```python
from build123d import *

# Parameters (mm, degrees)
BOSS_EXTRUDE1_DEPTH = 8.89
SKETCH3_R           = 3.556
BOSS_EXTRUDE2_DEPTH = 3.556


with BuildPart() as part:
    # Sketch2 → Boss-Extrude1 (new body)
    with BuildSketch(Plane.XY):
        with BuildLine():
            Line((-22.184810127, 0), (-33.106810127, 0))
            Line((-33.106810127, 0), (-33.106810127, 7.62))
            Line((-33.106810127, 7.62), (-25.486810127, 7.62))
            ThreePointArc((-25.486810127, 7.62), (-6.944810127, 22.300018764), (11.597189873, 7.62))
            Line((11.597189873, 7.62), (19.217189873, 7.62))
            Line((19.217189873, 7.62), (19.217189873, 0))
            Line((19.217189873, 0), (8.295189873, 0))
            ThreePointArc((8.295189873, 0), (-6.944810127, 15.24), (-22.184810127, 0))
        make_face()
    extrude(amount=BOSS_EXTRUDE1_DEPTH)

    # Sketch3 → Boss-Extrude2 (add)
    with BuildSketch(Plane.XZ):
        with Locations(Location((-27.645810127, 4.445, 0), (0, 0, 90))):
            Circle(SKETCH3_R)
        with Locations(Location((13.756189873, 4.445, 0), (0, 0, 90))):
            Circle(SKETCH3_R)
    extrude(amount=BOSS_EXTRUDE2_DEPTH)


solid = part.part
```
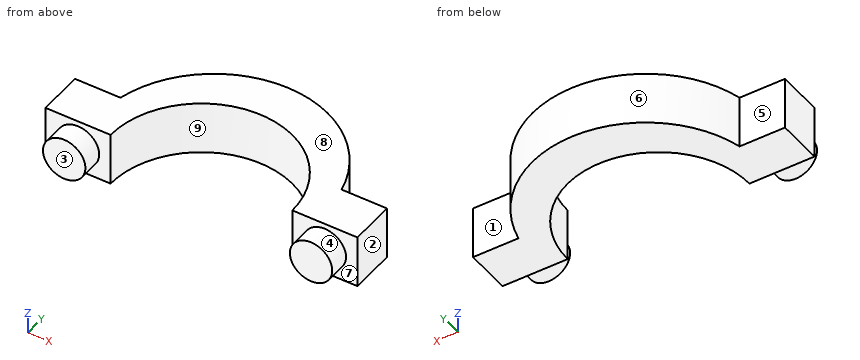
Geometry: final body of the model. Coordinates: model frame, mm. Face numbers are marked on the shaded views. A direction names the side the tool comes from. Round coordinates to 2 decimals unless told otherwise and drop trailing zeros. Write each loop counter-clockwise with the first axis right and the second up, starting at its lowest first coordinate (ties: lowest second). Pieces come first, ordered by that corner, then holes.
Item 1: Mould query, pull axis X, two halves, no side actions, for the marked faces 6, 7, 8 and 9. Classes: +X half, -X half, draft (parallel to the pull), parting line (faces both ways), or undercut.
Item 2: Section query C-C (y = 10). Return loops of the section in (x, z).
Item 3: Set-up query: the marked faces 1, 2, 3, 4 and 5. Return all of +Z, -Z, +X, -X, +Y, -Y with unobstructed straight access to the full face (end or side cutting, diameter ignored); none if empty.
Item 4: Material intervals for L1, parallel to X at y = -2, z = 6.5; L2, parallel to X at y = -2.5, z = 2.75; L3, parallel to Y at x = -28, z = 4.75, sorted ascending.
Item 5: Pin query (flat end, axial travel): P1, Ø4, axis at x = -28, z = 4, coming from the +Y side; P2, Ø8, axis at x = -3.5, y = 17, coming from the -Z side; P3, Ø3, axis at x = -8, y = 12, coming from the -Z side; P4, Ø4, axis at x = 10.5, z = 3, coming from the +Y side. Return the tip coordinate at first contact, or that it passes through.
Item 6: Section query A-A (y = 14). Return loops of the section in (x, z), plus the area to 3 significant figures.
Item 7: Section query B-B (z = 6.75). Return loops of the section in (x, y), plus the area to 3 significant figures.
Item 8: Section query D-D (x = -6). Return loops of the section in (y, z), plus the area to 3 significant figures.
Completed:
1. face 6: parting line
1. face 7: undercut
1. face 8: draft
1. face 9: undercut
2. outline: (-24.76, 0) - (-18.45, 0) - (-18.45, 8.89) - (-24.76, 8.89) - close; (4.56, 0) - (10.87, 0) - (10.87, 8.89) - (4.56, 8.89) - close
3. face 1: +Z, -Z, +X, +Y
3. face 2: +Z, -Z, +X, +Y, -Y
3. face 3: +Z, -Z, +X, -X, -Y
3. face 4: -Y
3. face 5: +Z, -Z, -X, +Y
4. L1: x = -30.55 to -24.74, 10.85 to 16.66
4. L2: x = -30.77 to -24.52, 10.63 to 16.88
4. L3: y = -3.56 to 7.62
5. P1: stops at y = 7.62
5. P2: stops at z = 0
5. P3: passes through
5. P4: stops at y = 14.4
6. outline: (-22.67, 0) - (-12.97, 0) - (-12.97, 8.89) - (-22.67, 8.89) - close; (-0.92, 0) - (8.78, 0) - (8.78, 8.89) - (-0.92, 8.89) - close
6. area: 173 mm2
7. outline: (-33.11, 0) - (-30.35, 0) - (-30.35, -3.56) - (-24.94, -3.56) - (-24.94, 0) - (-22.18, 0) arc R15.24 cw to (8.3, 0) - (11.05, 0) - (11.05, -3.56) - (16.46, -3.56) - (16.46, 0) - (19.22, 0) - (19.22, 7.62) - (11.6, 7.62) arc R19.05 ccw to (-25.49, 7.62) - (-33.11, 7.62) - close
7. area: 477 mm2
8. outline: (15.21, 0) - (22.28, 0) - (22.28, 8.89) - (15.21, 8.89) - close
8. area: 62.8 mm2
